The drawing under review shows one solid part. Ordinate dimensions are in mm from its lowest x, y, z. Coordinates: 2 decimals unless noted, no trailing zeros. Write each loop counter-clockwise with the first axis right and the second up, starting at its lowest first coordinate (ties: lowest second). Pieces come first, ordered by that corner, then holes.
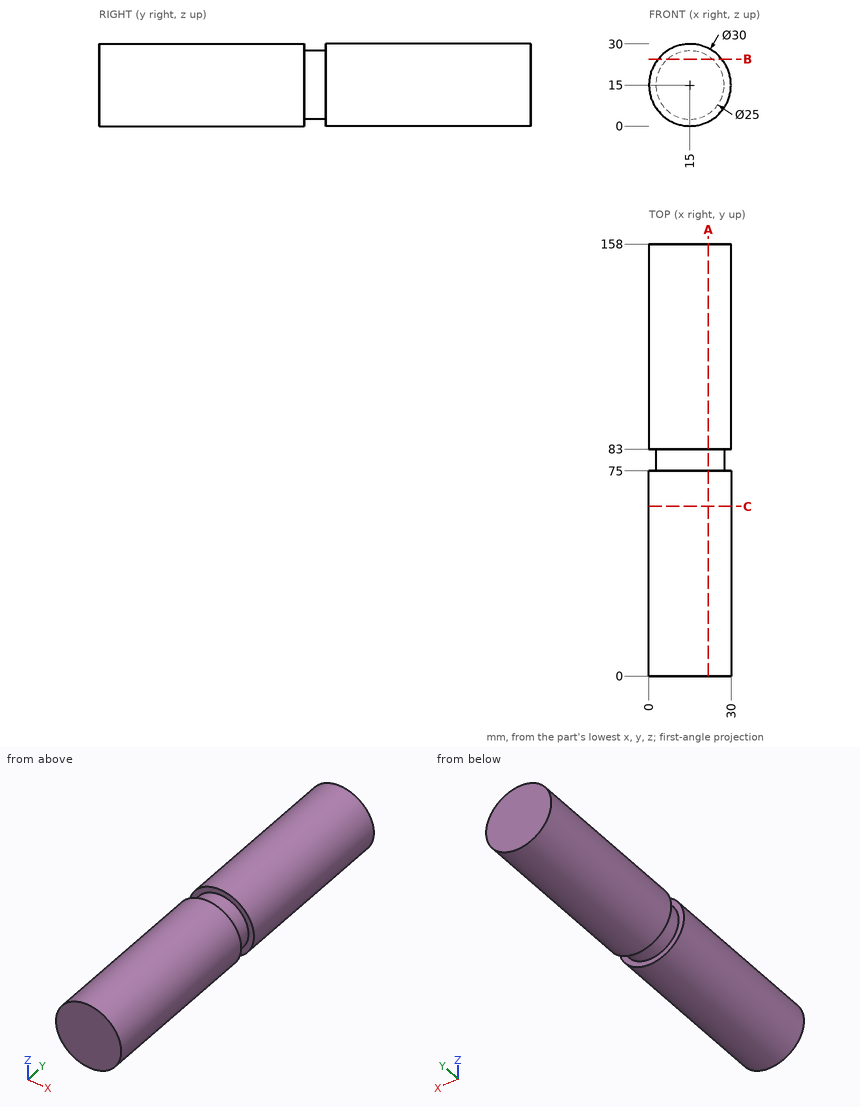
Q1. Clearance check with flat-ended pins moving along their axes: pin 1 Ø5 at (x, y) = (14.5, 53.5) entering from +Z; pin 2 Ø1.5 at (x, y) = (20.5, 24.5) entering from +Z; pin 3 Ø1 at (y, z) = (21, 25) entering from -X; pin 4 Ø8 at (y, z) = (81.5, 8.5) entering from +X. State where each tip first meets the part, or that it passes through.
Ans:
pin 1: stops at z = 30
pin 2: stops at z = 29.23
pin 3: stops at x = 3.39
pin 4: stops at x = 29.74
Q2. Add section B-B (z = 24.5). State the section outline as (x, y) points, then the cut area to 3 significant figures.
Ans:
outline: (3.39, 0) - (26.61, 0) - (26.61, 75) - (23.12, 75) - (23.12, 83) - (26.61, 83) - (26.61, 158) - (3.39, 158) - (3.39, 83) - (6.88, 83) - (6.88, 75) - (3.39, 75) - close
area: 3,610 mm2
Q3. Add section A-A (x = 21.75). State the section outline as (y, z) points.
Ans:
outline: (0, 1.6) - (75, 1.6) - (75, 4.48) - (83, 4.48) - (83, 1.6) - (158, 1.6) - (158, 28.4) - (83, 28.4) - (83, 25.52) - (75, 25.52) - (75, 28.4) - (0, 28.4) - close
Q4. For probe 1 along Y at (x, z) = (4, 21); probe 2 along X at (y, z) = (132.5, 14.75); probe 3 along X at (y, z) = (80, 18.5), list the stretches that pass through material, from the lowest coordinate up.
Ans:
probe 1: y = 0 to 75, 83 to 158
probe 2: x = 0 to 30
probe 3: x = 3 to 27
Q5. Add section C-C (y = 62). State the section outline as (x, z) points.
Ans:
outline: circle Ø30 at (15, 15)
